from build123d import *

# Parameters (mm, degrees)
SKETCH1_R               = 3.175
BOSS_EXTRUDE1_DEPTH     = 1.984375
SKETCH5_OUTSIDE_W       = 52.52
SKETCH5_OUTSIDE_H       = 54.24
SKETCH5_OUTSIDE_R       = 5.55625
CUT_EXTRUDE2_DEPTH      = 10.369388598
CUT_EXTRUDE2_DRAFT      = -60
MIRROR1_COPY_1_SKETCH_W = 52.52
MIRROR1_COPY_1_SKETCH_H = 54.24
MIRROR1_COPY_1_SKETCH_R = 5.55625
MIRROR1_COPY_1_DEPTH    = 10.369388598
MIRROR1_COPY_1_DRAFT    = -60


with BuildPart() as part:
    # Sketch1 → Boss-Extrude1 (new, symmetric)
    with BuildSketch(Plane(origin=(0, 0, 0), x_dir=(1, 0, 0), z_dir=(0, 1, 0))):
        Polygon((-5.55625, 3.207902433), (-5.55625, -3.207902433), (0, -6.415804866), (5.55625, -3.207902433), (5.55625, 3.207902433), (0, 6.415804866), align=None)
        with Locations(Location((0, 0, 0), (0, 0, 270))):
            Circle(SKETCH1_R, mode=Mode.SUBTRACT)
    extrude(amount=BOSS_EXTRUDE1_DEPTH, both=True)


with BuildPart() as cut_extrude2_tool:
    # Sketch5 outside → Cut-Extrude2 (with draft: the straight prism first)
    with BuildSketch(Plane(origin=(0, 1.984375, 0), x_dir=(1, 0, 0), z_dir=(0, 1, 0))):
        Rectangle(SKETCH5_OUTSIDE_W, SKETCH5_OUTSIDE_H)
        Circle(SKETCH5_OUTSIDE_R, mode=Mode.SUBTRACT)
    extrude(amount=-CUT_EXTRUDE2_DEPTH)
    # Cut-Extrude2: the draft: its side faces are tilted about the plane it starts from
    cut_extrude2_sides = [cut_extrude2_tool.faces().sort_by_distance(p)[0] for p in [
        (0, -3.200319299, 27.12),
        (26.26, -3.200319299, 0),
        (0, -3.200319299, -27.12),
        (-26.26, -3.200319299, 0),
        (-5.55625, -3.200319299, 0),
    ]]
    draft(cut_extrude2_sides, Plane(origin=(0, 1.984375, 0), x_dir=(1, 0, 0), z_dir=(0, 1, 0)), CUT_EXTRUDE2_DRAFT)


with BuildPart() as part_1:
    add(part.part)

    # Cut-Extrude2: cut by cut_extrude2_tool
    add(cut_extrude2_tool.part, mode=Mode.SUBTRACT)


with BuildPart() as mirror1_copy_1_tool:
    # Mirror1 copy 1 sketch → Mirror1 copy 1 (with draft: the straight prism first)
    with BuildSketch(Plane.XZ.offset(1.984375)):
        Rectangle(MIRROR1_COPY_1_SKETCH_W, MIRROR1_COPY_1_SKETCH_H)
        Circle(MIRROR1_COPY_1_SKETCH_R, mode=Mode.SUBTRACT)
    extrude(amount=-MIRROR1_COPY_1_DEPTH)
    # Mirror1 copy 1: the draft: its side faces are tilted about the plane it starts from
    mirror1_copy_1_sides = [mirror1_copy_1_tool.faces().sort_by_distance(p)[0] for p in [
        (0, 3.200319299, 27.12),
        (26.26, 3.200319299, 0),
        (0, 3.200319299, -27.12),
        (-26.26, 3.200319299, 0),
        (-5.55625, 3.200319299, 0),
    ]]
    draft(mirror1_copy_1_sides, Plane.XZ.offset(1.984375), MIRROR1_COPY_1_DRAFT)


with BuildPart() as part_2:
    add(part_1.part)

    # Mirror1 copy 1: cut by mirror1_copy_1_tool
    add(mirror1_copy_1_tool.part, mode=Mode.SUBTRACT)


solid = part_2.part
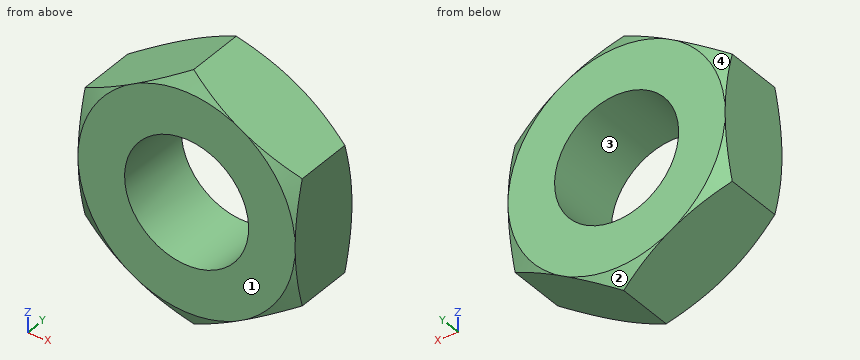
Source: CAD feature listing. Evaluate the final solid. Frame: model axes, mm. Face numbers are marked on the shaded views. Give positions to 0.01 mm unless a question says otherwise; leave off trailing zeros. Order: outer loops, then holes, each group sorted by start corner. A loop starts at its lowest first (then second) coordinate and runs counter-clockwise, first axis right, second up. Notation, with made-up numbers: (-9.5, 51.25) -> (30.5, 51.25) arc R21 cw to (30.5, 67.25) -> close; hole circle Ø6 at (14.25, 71). An arc over 180 degrees is marked (long way). Write item = value, one per line.
Q1. Material intervals for line 1 (X direction, y = 0.45, z = 0) (3 decimals); line 2 (X direction, y = -1.4, z = -1); line 3 (Z direction, x = 1.75, y = 0), sorted ascending. Write a range as from..to.
Data:
line_1 = -5.556..-3.175, 3.175..5.556
line_2 = -5.56..-3.01, 3.01..5.56
line_3 = -5.41..-2.65, 2.65..5.41
Q2. Cut plane A-A, the plane y = -0.15. Output: boundary loops of the cut face in (x, z) (3 decimals), and give its area (3 significant figures).
Data:
outline = (-5.556, -3.208) -> (0, -6.416) -> (5.556, -3.208) -> (5.556, 3.208) -> (0, 6.416) -> (-5.556, 3.208) -> close; hole circle Ø6.35 at (0, 0)
area = 75.3 mm^2
Q3. Pull-direction query (Z, two-part tool) for the marked faces 1, 2, 3 and 4; classes: released by +Z, released by -Z, zero draft, split by the parting line, or undercut.
Data:
face_1 = zero draft
face_2 = released by -Z
face_3 = undercut
face_4 = released by +Z
Q4. Cut plane B-B, the plane y = 1.7. Output: boundary loops of the cut face in (x, z) (3 decimals), and give its area (3 significant figures).
Data:
outline = (-5.556, -2.391) arc R6.049 ccw to (-4.849, -3.616) -> (-0.708, -6.007) arc R6.049 ccw to (0.708, -6.007) -> (4.849, -3.616) arc R6.049 ccw to (5.556, -2.391) -> (5.556, 2.391) arc R6.049 ccw to (4.849, 3.616) -> (0.708, 6.007) arc R6.049 ccw to (-0.708, 6.007) -> (-4.849, 3.616) arc R6.049 ccw to (-5.556, 2.391) -> close; hole circle Ø6.35 at (0, 0)
area = 73.8 mm^2
Q5. Pin query (flat end, axial travel): pin 1 (2 mm diameter, centred on x = -2, y = 0.5, fed in from -Z). Return the tip coordinate at first contact, or that it passes through.
Data:
pin_1 = -5.84
